```python
from build123d import *

# Parameters (mm, degrees)
PAD010_DEPTH    = 2
PAD013_DEPTH    = 2
SKETCH021_W     = 8
SKETCH021_H     = 11
SKETCH021_R     = 1.15
PAD014_DEPTH    = 5.5
FILLET003_R     = 6
FILLET006_R     = 1.99
SKETCH025_W     = 18
SKETCH025_H     = 5
POCKET008_DEPTH = 4
POCKET008_TAPER = 23


with BuildPart() as part:
    # Sketch014 → Pad010 (new body)
    with BuildSketch(Plane.XY):
        Polygon((-39, -15), (-15.75, -15), (-15.75, -22), (15.75, -22), (15.75, -15), (39, -15), (39, -51.5), (-39, -51.5), align=None)
    extrude(amount=PAD010_DEPTH)

    # Sketch020 (on Face10 of Pad010) → Pad013 (join)
    with BuildSketch(Plane.XY.offset(2)):
        Polygon((-14.5, -15.2), (-39.5, -15.2), (-39.5, -22.2), (39.378634, -22.2), (39.378634, -15.2), (14.378634, -15.2), (14.378634, -20.97266), (6.547439, -20.97266), (6.547439, -15.2), (3.839445, -15.2), (3.839445, -20.97266), (-3.90018, -20.97266), (-3.90018, -15.2), (-6.625733, -15.2), (-6.625733, -20.97266), (-14.5, -20.97266), align=None)
    extrude(amount=PAD013_DEPTH)

    # Sketch021 (on Face15 of Pad013) → Pad014 (join)
    with BuildSketch(Plane.XZ.offset(22.2)):
        with Locations((27.5, 8.9)):
            Rectangle(SKETCH021_W, SKETCH021_H)
        with Locations((27.5, 12.35)):
            Circle(SKETCH021_R, mode=Mode.SUBTRACT)
    extrude(amount=-PAD014_DEPTH)

    # Fillet003
    fillet003_edges = [part.edges().sort_by_distance(p)[0] for p in [
        (23.5, -19.45, 4),
        (31.5, -19.45, 4),
    ]]
    fillet(fillet003_edges, radius=FILLET003_R)

    # Fillet006
    fillet006_edges = [part.edges().sort_by_distance(p)[0] for p in [
        (0, -51.5, 0),
    ]]
    fillet(fillet006_edges, radius=FILLET006_R)

    # Sketch025 (on Face19 of Fillet006) → Pocket008 (cut)
    with BuildSketch(Plane.XY.offset(4)):
        with Locations((-26, -18.5)):
            Rectangle(SKETCH025_W, SKETCH025_H)
    extrude(amount=-POCKET008_DEPTH, taper=POCKET008_TAPER, mode=Mode.SUBTRACT)


solid = part.part
```
The model under review builds one solid part; all positions refer to its coordinate system, in mm. A direction names the side the tool comes from. Give positions to 0.01 mm unless a question says otherwise; leave off trailing zeros. Write each loop counter-clockwise with the first axis right and the second up, starting at its lowest first coordinate (ties: lowest second). Pieces come first, ordered by that corner, then holes.
(1) Consider section D-D, the plane y = -47. Give the boundary of the cut face in (x, z), and give its area (3 significant figures).
(2) The part is to be moulded in two halves that separate along X. For faces 5 (the flat face through (-27, -15.2, 3)), 6 (the flat face through (31.5, -19, 12)), 7 (the flat face through (-0.1, -21.4, 2)), say which applies: released by +X, released by -X, zero draft, split by the parting line, or undercut.
(3) To check wall thickness, follow L1, parallel to Z at x = 27.5, y = -18.8; L2, parallel to X at y = -29, z = 1.5; L3, parallel to Z at x = -2, y = -41. State the ranges of each line that lie inside material, in increasing order.
(4) Consider section B-B, the plane z = 12.35. Give the boundary of the cut face in (x, y), and give its area (4 significant figures).
(5) Tool access review of faces 1 (the flat face through (0, -20.973, 3)), 2 (the flat face through (1, -37, 2)), 3 (the flat face through (15.75, -19, 1)), 4 (the flat face through (27, -15.2, 3)): name each direction out of +Z, -Z, +X, -X, +Y, -Y from which nothing blocks a thin tool from reaching the whole face with its end or side.
(6) For P1, Ø1, axis at x = 0.5, z = 3, coming from the +Y side; P2, Ø1, axis at x = 21.5, z = 3, coming from the +Y side; P3, Ø8, axis at x = 8.5, y = -43.5, coming from the +Z side, all flat-tipped, find the tip position at first contact; note any pin that passes through.
Returned:
1. outline: (-39, 0) - (39, 0) - (39, 2) - (-39, 2) - close
1. area: 156 mm2
2. face 5: zero draft
2. face 6: released by +X
2. face 7: undercut
3. L1: z = 0 to 11.2, 13.5 to 14.4
3. L2: x = -39 to 39
3. L3: z = 0 to 2
4. outline: (23.5, -22.2) - (26.35, -22.2) - (26.35, -16.7) - (23.5, -16.7) - close; (28.65, -22.2) - (31.5, -22.2) - (31.5, -16.7) - (28.65, -16.7) - close
4. area: 31.35 mm2
5. face 1: +Z, -Z, +Y
5. face 2: +Z, +X, -X, -Y
5. face 3: -Z, +Y
5. face 4: +Z, +X, -X, +Y
6. P1: stops at y = -20.97
6. P2: stops at y = -15.2
6. P3: stops at z = 2
